Here's how the part is built. I have some questions about the finished solid (model axes, mm). Face numbers are marked on the shaded views. A direction names the side the tool comes from. Round coordinates to 2 decimals unless told otherwise and drop trailing zeros. Write each loop counter-clockwise with the first axis right and the second up, starting at its lowest first coordinate (ties: lowest second). Pieces come first, ordered by that corner, then holes. Notation, with made-up numbers: M 76,70.5 L 96,70.5 A19 cw 96,78.5 Z; hole C -35,11 d3. An arc over 180 degrees is marked long. Write item = value, one per line. Start each with the question number.
(1) I need wall thicknesses on line 1 along Z through (x, y) = (6, 4.5); line 2 along Y through (x, z) = (0.25, 25.5); line 3 along Z through (x, y) = (-1.75, 2.5). Which ranges of each line are inside material? Lowest first, please.
(2) Will these pins go through, and if not, where does the flat tip stop? pin 1 Ø4 at (x, z) = (-2.5, -0.5) entering from -Y; pin 2 Ø1.5 at (x, z) = (-1.5, 58.5) entering from +Y; pin 3 Ø1 at (x, z) = (5.5, 33.5) entering from -Y.
(3) I want a section at C-C (z = -8). List the corners of the cut face in (x, y) for me.
(4) On a 3-axis mill with a long thin cutter (end or side, diameter ignored), from which of +Z, -Z, +X, -X, +Y, -Y can I reach the whole of each face in a straight line? I mean the marked faces 1, 2 and 3. Say none if no direction works.
(5) I want a section at A-A (y = 0). List the corners of the cut face in (x, z) for me, and give its area (3 significant figures).
(6) I want a section at B-B (z = 44). List the corners of the cut face in (x, y) for me, and give its area (3 significant figures).
(7) I want a section at D-D (y = 8). List the corners of the cut face in (x, z) for me, and give its area (3 significant figures).
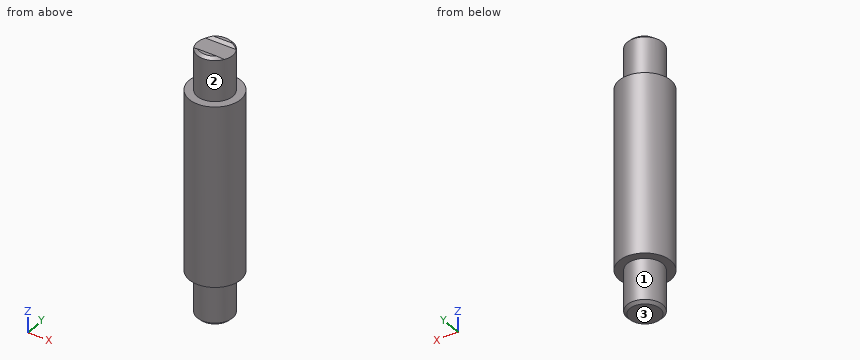
```python
from build123d import *

# Parameters (mm, degrees)
CROQUIS1_R              = 9.45
SALIENTE_EXTRUIR1_DEPTH = 66
CROQUIS7_R              = 6.5
SALIENTE_EXTRUIR5_DEPTH = 16
CHAFL_N5_SIZE           = 1
SALIENTE_EXTRUIR6_START = 16
CROQUIS12_R             = 6.5
SALIENTE_EXTRUIR6_DEPTH = 16
CORTAR_EXTRUIR12_DEPTH  = 1
CHAFL_N7_SIZE           = 1.25
CHAFL_N8_SIZE           = 1.25
CHAFL_N9_SIZE           = 1
CHAFL_N10_SIZE          = 1


with BuildPart() as part:
    # Croquis1 → Saliente-Extruir1 (new body)
    with BuildSketch(Plane.XY):
        Circle(CROQUIS1_R)
    extrude(amount=SALIENTE_EXTRUIR1_DEPTH)

    # Croquis7 → Saliente-Extruir5 (add)
    with BuildSketch(Plane(origin=(0, 0, 0), x_dir=(-1, 0, 0), z_dir=(0, 0, -1))):
        Circle(CROQUIS7_R)
    extrude(amount=SALIENTE_EXTRUIR5_DEPTH)

    # Chaflán5
    chafl_n5_edges = [part.edges().sort_by_distance(p)[0] for p in [
        (6.5, 0, -16),
    ]]
    chamfer(chafl_n5_edges, length=CHAFL_N5_SIZE)

    # Croquis12 → Saliente-Extruir6 (add)
    with BuildSketch(Plane.XY.offset(66).offset(SALIENTE_EXTRUIR6_START)):
        with Locations(Location((0, 0, 0), (0, 0, 180))):
            Circle(CROQUIS12_R)
    extrude(amount=-SALIENTE_EXTRUIR6_DEPTH)

    # Croquis13 → Cortar-Extruir12 (cut)
    with BuildSketch(Plane.XY.offset(82)):
        with BuildLine():
            Line((5.766281297, -3), (-5.766281297, -3))
            ThreePointArc((-5.766281297, -3), (-6.5, 0), (-5.766281297, 3))
            Line((-5.766281297, 3), (5.766281297, 3))
            ThreePointArc((5.766281297, 3), (6.5, 0), (5.766281297, -3))
        make_face()
    extrude(amount=-CORTAR_EXTRUIR12_DEPTH, mode=Mode.SUBTRACT)

    # Chaflán7
    # the kernel refuses this chamfer: 1.25 mm, written as the material it takes off along each edge
    with BuildSketch(Plane(origin=(-8.980885032, 3, 82), x_dir=(0, -0.02749587661058643, -0.9996219169112968), z_dir=(1, 0, 0))) as chafl_n7_piece_1_section:
        Polygon((CHAFL_N7_SIZE * 0.999621916911, CHAFL_N7_SIZE * 0.0274958766106), (-CHAFL_N7_SIZE * 0.0274958766106, CHAFL_N7_SIZE * 0.999621916911), (0, 0), align=None)
    chafl_n7_piece_1 = extrude(amount=17.961770065, mode=Mode.PRIVATE)
    chafl_n7_piece_1 = split(chafl_n7_piece_1, bisect_by=Plane(origin=(0, 3.432148015, 81), z_dir=(0, 0, 1)), keep=Keep.TOP, mode=Mode.PRIVATE)
    add(chafl_n7_piece_1, mode=Mode.SUBTRACT)

    # Chaflán8
    # the kernel refuses this chamfer: 1.25 mm, written as the material it takes off along each edge
    with BuildSketch(Plane(origin=(8.980885032, -3, 82), x_dir=(0, -0.9996219169112969, 0.027495876610582178), z_dir=(-1, 0, 0))) as chafl_n8_piece_1_section:
        Polygon((CHAFL_N8_SIZE * 0.999621916911, -CHAFL_N8_SIZE * 0.0274958766106), (-CHAFL_N8_SIZE * 0.0274958766106, -CHAFL_N8_SIZE * 0.999621916911), (0, 0), align=None)
    chafl_n8_piece_1 = extrude(amount=17.961770065, mode=Mode.PRIVATE)
    chafl_n8_piece_1 = split(chafl_n8_piece_1, bisect_by=Plane(origin=(0, -3.432148015, 81), z_dir=(0, 0, 1)), keep=Keep.TOP, mode=Mode.PRIVATE)
    add(chafl_n8_piece_1, mode=Mode.SUBTRACT)

    # Chaflán9
    chafl_n9_edges = [part.edges().sort_by_distance(p)[0] for p in [
        (0, 6.5, 82),
    ]]
    chamfer(chafl_n9_edges, length=CHAFL_N9_SIZE)

    # Chaflán10
    chafl_n10_edges = [part.edges().sort_by_distance(p)[0] for p in [
        (0, -6.5, 82),
    ]]
    chamfer(chafl_n10_edges, length=CHAFL_N10_SIZE)


solid = part.part
```
Returned:
q1.line_1 = 0 to 66
q1.line_2 = -9.45 to 9.45
q1.line_3 = -16 to 81
q2.pin_1 = -9.43
q2.pin_2 = 9.42
q2.pin_3 = -8.02
q3.outline = C 0,0 d13
q4.face_1 = -Z
q4.face_2 = +Z
q4.face_3 = -Z, +X, -X, +Y, -Y
q5.outline = M -9.45,0 L -6.5,0 L -6.5,-15 L -5.5,-16 L 5.5,-16 L 6.5,-15 L 6.5,0 L 9.45,0 L 9.45,66 L 6.5,66 L 6.5,81 L -6.5,81 L -6.5,66 L -9.45,66 Z
q5.area = 1,650 mm²
q6.outline = C 0,0 d18.9
q6.area = 281 mm²
q7.outline = M -5.03,0 L 5.03,0 L 5.03,66 L -5.03,66 Z
q7.area = 664 mm²
